Could you check a few things on this drawing? It's one solid part, dimensions in mm from its lowest x, y, z. A direction names the side the tool comes from. Give positions to 0.01 mm unless a question says otherwise; leave off trailing zeros. Order: outer loops, then holes, each group sorted by start corner. A loop starts at its lowest first (then second) coordinate and runs counter-clockwise, first axis right, second up. Notation, with made-up numbers: (-30, 48) -> (24, 48) arc R24 cw to (24, 76) -> close; hole circle Ø8 at (-14.75, 68.5). An arc over 180 degrees is marked (long way). Write each question's results on one line, items separated by ' | '. Start each with the question number.
Q1. I'm going to push a flat-ended pin straight in: pin 1 (10 mm diameter, centred on x = 67.5, y = 12, fed in from +Z). Where does the tip first touch, or does it pass through?
Q2. Thinking about a two-plate mould opening in Y: for the marked faces 1, 2 and 3, which applies, pulls with the +Y half, pulls with the -Y half, needs draft (parallel to the pull), parting line crosses it, or undercut?
Q3. Imagine slicing it at C-C, the plane x = 17.5. Please give me the cut outline in (y, z).
Q4. For the marked faces 4 and 5, which set-ups out of +Z, -Z, +X, -X, +Y, -Y let a thin tool reach every point of the face, with its end or its side?
Q5. Imagine slicing it at A-A, the plane y = 12. Please give me the cut outline in (x, z).
Q6. Imagine slicing it at B-B, the plane z = 12.5. Please give me the cut outline in (x, y).
Q7. I need wall thicknesses on line 1 along Y through (x, z) = (67.5, 6); line 2 along X through (y, z) = (12, 8.25); line 3 along Y through (x, z) = (42.5, 6.5). Which ranges of each line are inside material? Lowest first, please. Write a range as [from, to].
Q8. Imagine slicing it at D-D, the plane y = 7.75. Please give me the cut outline in (x, z).
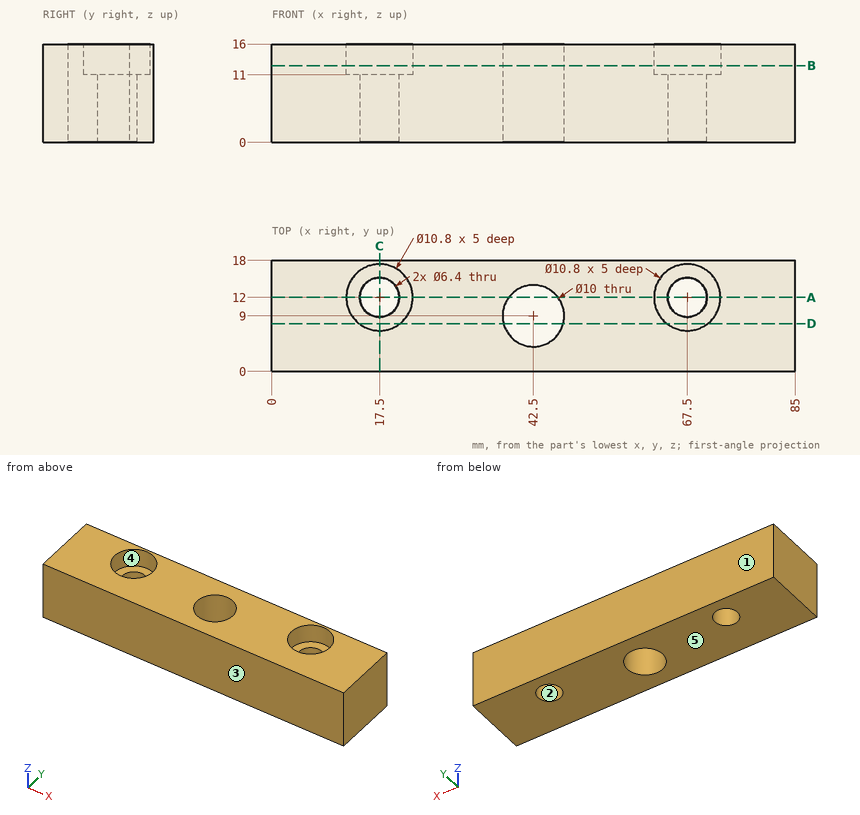
Geometry check:
1) pin 1: z = 11
2) face 1: pulls with the +Y half | face 2: undercut | face 3: pulls with the -Y half
3) outline: (0, 0) -> (8.8, 0) -> (8.8, 11) -> (6.6, 11) -> (6.6, 16) -> (0, 16) -> close; (15.2, 0) -> (18, 0) -> (18, 16) -> (17.4, 16) -> (17.4, 11) -> (15.2, 11) -> close
4) face 4: +Z | face 5: -Z, +X, -X, +Y, -Y
5) outline: (0, 0) -> (14.3, 0) -> (14.3, 11) -> (12.1, 11) -> (12.1, 16) -> (0, 16) -> close; (20.7, 0) -> (38.5, 0) -> (38.5, 16) -> (22.9, 16) -> (22.9, 11) -> (20.7, 11) -> close; (46.5, 0) -> (64.3, 0) -> (64.3, 11) -> (62.1, 11) -> (62.1, 16) -> (46.5, 16) -> close; (70.7, 0) -> (85, 0) -> (85, 16) -> (72.9, 16) -> (72.9, 11) -> (70.7, 11) -> close
6) outline: (0, 0) -> (85, 0) -> (85, 18) -> (0, 18) -> close; hole circle Ø10.8 at (17.5, 12); hole circle Ø10 at (42.5, 9); hole circle Ø10.8 at (67.5, 12)
7) line 1: [0, 8.8], [15.2, 18] | line 2: [0, 14.3], [20.7, 38.5], [46.5, 64.3], [70.7, 85] | line 3: [0, 4], [14, 18]
8) outline: (0, 0) -> (37.66, 0) -> (37.66, 16) -> (20.83, 16) -> (20.83, 11) -> (14.17, 11) -> (14.17, 16) -> (0, 16) -> close; (47.34, 0) -> (85, 0) -> (85, 16) -> (70.83, 16) -> (70.83, 11) -> (64.17, 11) -> (64.17, 16) -> (47.34, 16) -> close
